Design review of the part built by this model. Coordinates are the model's own, in mm. Round coordinates to 2 decimals unless told otherwise and drop trailing zeros. Loops run counter-clockwise (first coordinate to the right, second up) from the corner with the lowest first, then second, coordinate; pieces in that order, holes last. Notation, with made-up numbers: (-17.5, 69) - (-1.5, 69) arc R36 cw to (-1.5, 103) - close; hole circle Ø5 at (67, 5.5). An arc over 180 degrees is marked (long way). Return JSON: item names as keys, results as strings. Group by question number.
from build123d import *

# Parameters (mm, degrees)
EXTRUDE_1_DEPTH = 2.75


with BuildPart() as part:
    # 草图1 → 凸台-拉伸1 (new body)
    with BuildSketch(Plane.XY):
        Polygon((200, 0), (200, 27), (200, 30), (195, 30), (195, 33), (200, 33), (200, 230), (200, 232.75), (195, 232.75), (195, 230), (5, 230), (5, 232.75), (0, 232.75), (0, 230), (0, 33), (5, 33), (5, 30), (0, 30), (0, 27), (0, 0), (4, 0), (4, -3), (10, -3), (10, 0), (29, 0), (29, 5), (71, 5), (71, 0), (41, 0), (41, -3), (159, -3), (159, 0), (129, 0), (129, 5), (171, 5), (171, 0), (190, 0), (190, -3), (196, -3), (196, 0), align=None)
        Polygon((95, 5), (100, 5), (105, 5), (105, 20), (95, 20), align=None, mode=Mode.SUBTRACT)
    extrude(amount=EXTRUDE_1_DEPTH)


solid = part.part
Q1. For line 1 (Y direction, x = 65, z = 0.7); line 2 (Y direction, x = 102, z = 2.25); line 3 (Y direction, x = 181, z = 0.5), list the stretches that pass through material, from the lowest coordinate up.
Q2. Insertion check: pin 1 Ø1 at (x, y) = (158.5, 146.5) entering from -Z; pin 2 Ø1.4 at (y, z) = (32, 2) entering from -X; pin 3 Ø0.8 at (x, z) = (198.5, 1.5) entering from -Y. Each pin has a flat end and moves straight along its axis. Give the tip position at first contact, or say it passes through.
Q3. Add section B-B, the plane x = 26.5. State the section outline as (y, z) points.
Q4. Add section A-A, the plane x = 58.5. State the section outline as (y, z) points, plus the area to 3 significant figures.
Evaluation:
{
 "1": {"line 1": "-3 to 0, 5 to 230", "line 2": "-3 to 5, 20 to 230", "line 3": "0 to 230"},
 "2": {"pin 1": "z = 0", "pin 2": "x = 5", "pin 3": "y = 0"},
 "3": {"outline": "(0, 0) - (230, 0) - (230, 2.75) - (0, 2.75) - close"},
 "4": {"outline": "(-3, 0) - (0, 0) - (0, 2.75) - (-3, 2.75) - close; (5, 0) - (230, 0) - (230, 2.75) - (5, 2.75) - close", "area": "627 mm²"}
}
